from build123d import *

# Parameters (mm, degrees)
SKETCH1_W           = 70
SKETCH1_H           = 70
SKETCH1_W_2         = 60
SKETCH1_H_2         = 60
BOSS_EXTRUDE1_DEPTH = 15
BOSS_EXTRUDE2_START = 15
SKETCH1_2_W         = 70
SKETCH1_2_H         = 70
BOSS_EXTRUDE2_DEPTH = 2
CUT_EXTRUDE1_DEPTH  = 53.5
CUT_EXTRUDE2_DEPTH  = 38.5
CUT_EXTRUDE3_START  = 13
SKETCH4_W           = 34
SKETCH4_H           = 42
CUT_EXTRUDE3_DEPTH  = 5
FILLET1_R           = 3.6
SKETCH5_R           = 1.6
CUT_EXTRUDE4_DEPTH  = 25
SKETCH7_W           = 60
SKETCH7_H           = 5
CUT_EXTRUDE5_DEPTH  = 1.6


with BuildPart() as part:
    # Sketch1 → Boss-Extrude1 (new body)
    with BuildSketch(Plane(origin=(0, 0, 0), x_dir=(1, 0, 0), z_dir=(0, 1, 0))):
        Rectangle(SKETCH1_W, SKETCH1_H)
        Rectangle(SKETCH1_W_2, SKETCH1_H_2, mode=Mode.SUBTRACT)
    extrude(amount=BOSS_EXTRUDE1_DEPTH)

    # Sketch1<2> → Boss-Extrude2 (add)
    with BuildSketch(Plane(origin=(0, 0, 0), x_dir=(1, 0, 0), z_dir=(0, 1, 0)).offset(BOSS_EXTRUDE2_START)):
        Rectangle(SKETCH1_2_W, SKETCH1_2_H)
    extrude(amount=-BOSS_EXTRUDE2_DEPTH)

    # Sketch2 → Cut-Extrude1 (cut, symmetric)
    with BuildSketch(Plane.XY):
        with BuildLine():
            Line((-15, 11), (15, 11))
            ThreePointArc((15, 11), (18, 8), (15, 5))
            Line((15, 5), (-15, 5))
            ThreePointArc((-15, 5), (-18, 8), (-15, 11))
        make_face()
    extrude(amount=CUT_EXTRUDE1_DEPTH, both=True, mode=Mode.SUBTRACT)

    # Sketch3 → Cut-Extrude2 (cut, symmetric)
    with BuildSketch(Plane(origin=(0, 0, 0), x_dir=(0, 0, -1), z_dir=(1, 0, 0))):
        with BuildLine():
            Line((15, 5), (-15, 5))
            ThreePointArc((-15, 5), (-18, 8), (-15, 11))
            Line((-15, 11), (15, 11))
            ThreePointArc((15, 11), (18, 8), (15, 5))
        make_face()
    extrude(amount=CUT_EXTRUDE2_DEPTH, both=True, mode=Mode.SUBTRACT)

    # Sketch4 → Cut-Extrude3 (cut)
    with BuildSketch(Plane(origin=(0, 0, 0), x_dir=(1, 0, 0), z_dir=(0, 1, 0)).offset(CUT_EXTRUDE3_START)):
        Rectangle(SKETCH4_W, SKETCH4_H)
    extrude(amount=CUT_EXTRUDE3_DEPTH, mode=Mode.SUBTRACT)

    # Fillet1
    fillet1_edges = [part.edges().sort_by_distance(p)[0] for p in [
        (17, 14, 21),
        (17, 14, -21),
        (-17, 14, -21),
        (-17, 14, 21),
    ]]
    fillet(fillet1_edges, radius=FILLET1_R)

    # Sketch5 → Cut-Extrude4 (cut)
    with BuildSketch(Plane(origin=(0, 0, 0), x_dir=(1, 0, 0), z_dir=(0, 1, 0))):
        with Locations((-23.75, 32.5)):
            Circle(SKETCH5_R)
        with Locations((-23.75, -32.5)):
            Circle(SKETCH5_R)
        with Locations((23.75, 32.5)):
            Circle(SKETCH5_R)
        with Locations((23.75, -32.5)):
            Circle(SKETCH5_R)
    extrude(amount=CUT_EXTRUDE4_DEPTH, mode=Mode.SUBTRACT)

    # Sketch7 → Cut-Extrude5 (cut)
    with BuildSketch(Plane(origin=(0, 0, 0), x_dir=(1, 0, 0), z_dir=(0, 1, 0))):
        with Locations((0, 32.5)):
            Rectangle(SKETCH7_W, SKETCH7_H)
        with Locations((0, -32.5)):
            Rectangle(SKETCH7_W, SKETCH7_H)
    extrude(amount=CUT_EXTRUDE5_DEPTH, mode=Mode.SUBTRACT)


solid = part.part
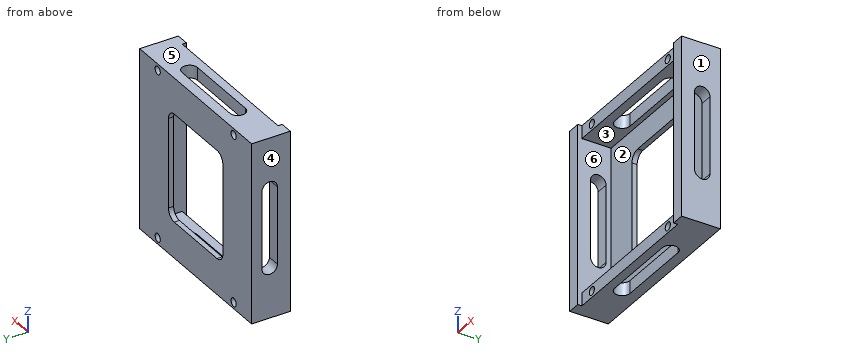
Verification items for the finished model (mm, model axes). Face numbers are marked on the shaded views. A direction names the side the tool comes from. Give positions to 0.01 mm unless a question says otherwise; leave off trailing zeros. Order: outer loops, then holes, each group sorted by start corner. A loop starts at its lowest first (then second) coordinate and runs counter-clockwise, first axis right, second up. Notation, with made-up numbers: (81, 42.25) -> (136, 42.25) arc R28 ccw to (136, 78.25) -> close; hole circle Ø10 at (35.25, 49). An arc over 180 degrees is marked (long way). Answer as CSV lines item,"result".
Q1. Sectioned sample at C-C on y = 8. Record the cut outline in (x, z).
Solutions:
outline,"(-35, -35) -> (-18, -35) -> (-18, -30) -> (-30, -30) -> (-30, -18) -> (-35, -18) -> close; (-35, 18) -> (-30, 18) -> (-30, 30) -> (-18, 30) -> (-18, 35) -> (-35, 35) -> close; (18, -35) -> (35, -35) -> (35, -18) -> (30, -18) -> (30, -30) -> (18, -30) -> close; (18, 30) -> (30, 30) -> (30, 18) -> (35, 18) -> (35, 35) -> (18, 35) -> close; hole circle Ø3.2 at (-23.75, -32.5); hole circle Ø3.2 at (-23.75, 32.5); hole circle Ø3.2 at (23.75, -32.5); hole circle Ø3.2 at (23.75, 32.5)"
Q2. Scan lines: probe 1 along Z at (x, y) = (-23.75, 8.5); probe 2 along X at (y, z) = (13.5, 15); probe 3 along X at (y, z) = (3.5, 13.5). Record each from-to range of solid material in increasing order.
Solutions:
probe 1,"z = -35 to -34.1, -30.9 to -30, 30 to 30.9, 34.1 to 35"
probe 2,"x = -35 to -17, 17 to 35"
probe 3,"x = -35 to -30, 30 to 35"
Q3. Depth check by flat-ended pin: pin 1 (3 mm diameter, centred on x = 14.5, z = 25.5, fed in from -Y); pin 2 (1.5 mm diameter, centred on x = 3.5, z = 31.5, fed in from -Y); pin 3 (3 mm diameter, centred on x = 0.5, y = 9, fed in from -Z). Enter the tip coordinate at first touch or a pass-through.
Solutions:
pin 1,"stops at y = 13"
pin 2,"stops at y = 1.6"
pin 3,"passes through"
Q4. Sectioned sample at D-D on z = 7.5. Record the cut outline in (x, y), plus the area to 3 significant figures.
Solutions:
outline,"(-35, 0) -> (-30, 0) -> (-30, 5) -> (-35, 5) -> close; (-35, 11) -> (-30, 11) -> (-30, 13) -> (-17, 13) -> (-17, 15) -> (-35, 15) -> close; (17, 13) -> (30, 13) -> (30, 11) -> (35, 11) -> (35, 15) -> (17, 15) -> close; (30, 0) -> (35, 0) -> (35, 5) -> (30, 5) -> close"
area,"142 mm²"
Q5. Sectioned sample at B-B on x = -23.75. Record the cut outline in (y, z).
Solutions:
outline,"(1.6, -35) -> (15, -35) -> (15, -34.1) -> (1.6, -34.1) -> close; (1.6, -30.9) -> (15, -30.9) -> (15, 30.9) -> (1.6, 30.9) -> (1.6, 30) -> (13, 30) -> (13, -30) -> (1.6, -30) -> close; (1.6, 34.1) -> (15, 34.1) -> (15, 35) -> (1.6, 35) -> close"
Q6. Sectioned sample at A-A on z = -32.5. Record the cut outline in (x, y), plus the area to 3 significant figures.
Solutions:
outline,"(-35, 0) -> (-30, 0) -> (-30, 1.6) -> (-25.35, 1.6) -> (-25.35, 15) -> (-35, 15) -> close; (-22.15, 1.6) -> (22.15, 1.6) -> (22.15, 15) -> (-22.15, 15) -> close; (25.35, 1.6) -> (30, 1.6) -> (30, 0) -> (35, 0) -> (35, 15) -> (25.35, 15) -> close; hole (-15, 5) -> (15, 5) arc R3 ccw to (15, 11) -> (-15, 11) arc R3 ccw to start"
area,"660 mm²"
Q7. Access from +Z, -Z, +X, -X, +Y, -Y to the whole of each face (thin tool, end or side, straight path). Record for the marked faces 1 and 2.
Solutions:
face 1,"+Z, -Z, +X, +Y, -Y"
face 2,"-Y"
Q8. Release check for a two-part mould opening along Z. For the marked faces 3, 4, 5 and 6 record: +Z half, -Z half, draft (parallel to the pull), parting line (faces both ways), or undercut.
Solutions:
face 3,"undercut"
face 4,"draft"
face 5,"+Z half"
face 6,"undercut"
